Check sheet for the modelled part. Datum: model origin and axes. Units: mm. Face numbers are marked on the shaded views. A direction names the side the tool comes from. Give positions to 0.01 mm unless a question says otherwise; leave off trailing zeros. Loops run counter-clockwise (first coordinate to the right, second up) from the corner with the lowest first, then second, coordinate; pieces in that order, holes last. Notation, with made-up numbers: (9.5, 32) - (41.5, 32) arc R23 ccw to (41.5, 63) - close; hole circle Ø5 at (-6, 54.25). An arc over 180 degrees is marked (long way). Answer in a Markdown table with one row per item. Add a question column.
(1) Sectioned sample at C-C on y = 22. Enter the section's corners in (x, z).
(2) Sectioned sample at B-B on z = -11.5. Enter the section's corners in (x, y).
(3) Sectioned sample at A-A on y = 10.5. Enter the section's corners in (x, z).
(4) Go/stop test with flat-tipped pins: P1, Ø12, axis at x = 8, z = -13, coming from the +Y side; P2, Ø7, axis at x = 10.5, y = 8, coming from the -Z side; P3, Ø11, axis at x = 10.5, z = -16.5, coming from the -Y side. Record where each tip stops, or that it passes through.
(5) Sectioned sample at D-D on x = 14.75. Enter the section's corners in (y, z).
(6) Set-up check for the marked faces 1 and 2: record each of +Z, -Z, +X, -X, +Y, -Y from which the full face is reachable in a straight line by a thin tool's end or side.
(7) Thickness scan on L1, parallel to X at y = 23.5, z = -6.75; L2, parallel to Y at x = 8, z = -26; L3, parallel to Z at x = 4.5, y = 4.25. Record the ranges inside material, lowest first.
(8) Draft check along X on the marked faces 3, 4 and 5. Enter one of: released by +X, released by -X, zero draft, split by the parting line, or undercut.
Autodesk Inventor part; units mm, degrees
ref_plane "YZ Plane" through (0, 0, 0) normal (1, 0, 0) x (0, 1, 0)
ref_plane "XZ Plane" through (0, 0, 0) normal (0, 1, 0) x (-1, 0, 0)
ref_plane "XY Plane" through (0, 0, 0) normal (0, 0, 1) x (1, 0, 0)
sketch "Boceto1" plane through (0, 0, 0) normal (1, 0, 0) x (0, 1, 0)
  line L0 (0, 0) -> (28, 0)
  line L1 (28, 0) -> (28, -28)
  line L2 (28, -28) -> (24, -28)
  line L3 (24, -28) -> (24, -4)
  line L4 (24, -4) -> (0, -4)
  line L5 (0, -4) -> (0, 0)
  dimension "d0" = 28
  dimension "d1" = 28
  dimension "d2" = 4
  dimension "d3" = 4
extrude "Extrusión1" add sketch "Boceto1" along normal blind 20
sketch "Boceto4" plane through (20, 0, 0) normal (1, 0, 0) x (0, 0, -1)
  line L0 (4, 24) -> (28, 24)
  line L1 (4, 0) -> (4, 24)
  line L2 (28, 24) -> (28, 28)
  line L3 (28, 24) -> (28, 21.5)
  line L4 (28, 21.5) -> (6.5, 0)
  line L5 (0, 0) -> (4, 0)
  line L6 (6.5, 0) -> (4, 0)
  dimension "d21" = 45
  dimension "d22" = 2.5
extrude "Extrusión4" add sketch "Boceto4" against normal blind 3
sketch "Boceto5" plane through (0, 0, 0) normal (-1, 0, 0) x (0, 0, 1)
  line L0 (-28, 24) -> (-28, 21.5)
  line L1 (-28, 21.5) -> (-6.5, 0)
  line L2 (-6.5, 0) -> (-4, 0)
  line L3 (-4, 24) -> (-4, 0)
  line L4 (-28, 24) -> (-4, 24)
  point P0 (0, 0)
extrude "Extrusión5" add sketch "Boceto5" against normal blind 3
sketch "Boceto6" plane through (17, 24, -28) normal (0, -1, 0) x (1, 0, 0)
  line L0 (-14, 24) -> (0, 24)
  line L1 (-14, 24) -> (0, 24)
  line L2 (-7, 24) -> (-7, 0) construction
  line L3 (-14, 0) -> (0, 0)
  circle A0 centre (-7, 18) radius 2
  circle A1 centre (-7, 8) radius 2
  line L4 (-17, 28) -> (3, 28)
  line L5 (-9, 18) -> (-9, 8)
  line L6 (-5, 8) -> (-5, 18)
  dimension "d27" = 10
  dimension "d28" = 4
  dimension "d29" = 4
  dimension "d30" = 10
extrude "Extrusión6" cut sketch "Boceto6" against normal through all
fillet "Empalme4" radius 1 8 edges at (10, 24, -22) (8, 24, -15) (10, 24, -8) (12, 24, -15) (10, 28, -8) (8, 28, -15) (10, 28, -22) (12, 28, -15)
sketch "Boceto7" plane through (17, 0, -4) normal (0, 0, -1) x (-1, 0, 0)
  circle A0 centre (7, 8) radius 2
  circle A1 centre (7, 18) radius 2
  line L0 (14, 0) -> (0, 0)
  line L1 (9, 18) -> (9, 8)
  line L2 (5, 18) -> (5, 8)
  line L3 (17, 0) -> (-3, 0)
  line L4 (7, 0) -> (7, 24) construction
  line L5 (14, 24) -> (0, 24)
  dimension "d34" = 4
  dimension "d35" = 4
  dimension "d36" = 10
  dimension "d37" = 8
extrude "Extrusión7" cut sketch "Boceto7" against normal through all
fillet "Empalme5" radius 1 8 edges at (8, 13, -4) (10, 6, -4) (12, 13, -4) (10, 20, -4) (10, 20, 0) (12, 13, 0) (10, 6, 0) (8, 13, 0)
properties part number "Angulo S" material "Aluminio 6061"
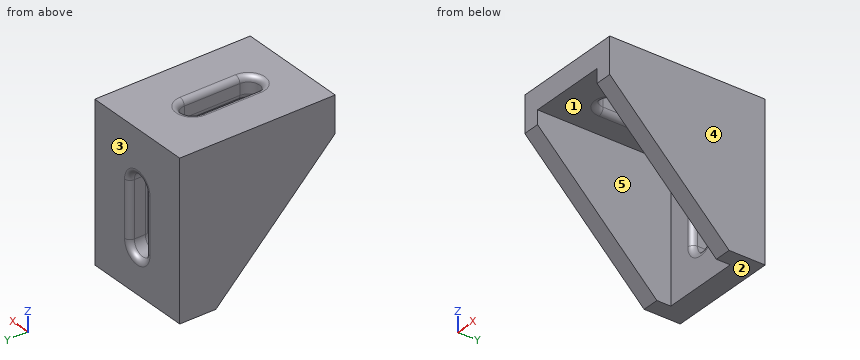
Reply:
| question | item | result |
|---|---|---|
| 1 | outline | (0, -28) - (3, -28) - (3, -4) - (17, -4) - (17, -28) - (20, -28) - (20, 0) - (0, 0) - close |
| 2 | outline | (0, 5) - (3, 5) - (3, 24) - (7, 24) arc R1 ccw to (8, 25) - (8, 27) arc R1 ccw to (7, 28) - (0, 28) - close; (12, 25) arc R1 ccw to (13, 24) - (17, 24) - (17, 5) - (20, 5) - (20, 28) - (13, 28) arc R1 ccw to (12, 27) - close |
| 3 | outline | (0, -17) - (3, -17) - (3, -4) - (7, -4) arc R1 ccw to (8, -3) - (8, -1) arc R1 ccw to (7, 0) - (0, 0) - close; (12, -3) arc R1 ccw to (13, -4) - (17, -4) - (17, -17) - (20, -17) - (20, 0) - (13, 0) arc R1 ccw to (12, -1) - close |
| 4 | P1 | y = 28 |
| 4 | P2 | z = -4 |
| 4 | P3 | y = 24 |
| 5 | outline | (0, -4) - (24, -4) - (24, -28) - (28, -28) - (28, 0) - (0, 0) - close |
| 6 | face 1 | -Z, -Y |
| 6 | face 2 | -Z, +X, -X, +Y, -Y |
| 7 | L1 | 0 to 3, 17 to 20 |
| 7 | L2 | 24 to 28 |
| 7 | L3 | -4 to 0 |
| 8 | face 3 | zero draft |
| 8 | face 4 | released by +X |
| 8 | face 5 | undercut |
